from build123d import *

# Parameters (mm, degrees)
SKETCH1_R           = 15
BOSS_EXTRUDE1_DEPTH = 5
SKETCH2_R           = 19
SKETCH2_R_2         = 15
BOSS_EXTRUDE2_DEPTH = 40
SKETCH3_R           = 5
SKETCH3_R_2         = 15
BOSS_EXTRUDE4_DEPTH = 5
BOSS_EXTRUDE5_REACH = 62
SKETCH4_R           = 19
SKETCH5_R           = 10
CUT_EXTRUDE1_DEPTH  = 10
SKETCH6_R           = 5
CUT_EXTRUDE2_DEPTH  = 48
BOSS_EXTRUDE6_REACH = 62
SKETCH7_R           = 6
SKETCH8_R           = 2
CUT_EXTRUDE3_DEPTH  = 15


with BuildPart() as part:
    # Sketch1 → Boss-Extrude1 (new body)
    with BuildSketch(Plane(origin=(0, 0, 0), x_dir=(1, 0, 0), z_dir=(0, 1, 0))):
        with BuildLine():
            Line((-9.090909091, 17.814470857), (-30.909090909, 6.680426571))
            ThreePointArc((-30.909090909, 6.680426571), (-35, 0), (-30.909090909, -6.680426571))
            Line((-30.909090909, -6.680426571), (-9.090909091, -17.814470857))
            ThreePointArc((-9.090909091, -17.814470857), (0, -20), (9.090909091, -17.814470857))
            Line((9.090909091, -17.814470857), (30.909090909, -6.680426571))
            ThreePointArc((30.909090909, -6.680426571), (35, 0), (30.909090909, 6.680426571))
            Line((30.909090909, 6.680426571), (9.090909091, 17.814470857))
            ThreePointArc((9.090909091, 17.814470857), (0, 20), (-9.090909091, 17.814470857))
        make_face()
        Circle(SKETCH1_R, mode=Mode.SUBTRACT)
        with BuildLine():
            Line((-23.5, 2), (-24.035898385, 2))
            ThreePointArc((-24.035898385, 2), (-31.5, 0), (-24.035898385, -2))
            Line((-24.035898385, -2), (-23.5, -2))
            Line((-23.5, -2), (-19.5, -2))
            Line((-19.5, -2), (-19.5, 2))
            Line((-19.5, 2), (-23.5, 2))
        make_face(mode=Mode.SUBTRACT)
        with BuildLine():
            Line((23.5, 2), (24.035898385, 2))
            ThreePointArc((24.035898385, 2), (31.5, 0), (24.035898385, -2))
            Line((24.035898385, -2), (23.5, -2))
            Line((23.5, -2), (19.5, -2))
            Line((19.5, -2), (19.5, 2))
            Line((19.5, 2), (23.5, 2))
        make_face(mode=Mode.SUBTRACT)
    extrude(amount=BOSS_EXTRUDE1_DEPTH)

    # Sketch2 → Boss-Extrude2 (add)
    with BuildSketch(Plane(origin=(0, 5, 0), x_dir=(1, 0, 0), z_dir=(0, 1, 0))):
        Circle(SKETCH2_R)
        Circle(SKETCH2_R_2, mode=Mode.SUBTRACT)
    extrude(amount=BOSS_EXTRUDE2_DEPTH)

    # Sketch3 → Boss-Extrude4 (add)
    with BuildSketch(Plane(origin=(0, 45, 0), x_dir=(1, 0, 0), z_dir=(0, 1, 0))):
        with BuildLine():
            Line((9.090909091, -17.814470857), (30.909090909, -6.680426571))
            ThreePointArc((30.909090909, -6.680426571), (35, 0), (30.909090909, 6.680426571))
            Line((30.909090909, 6.680426571), (9.090909091, 17.814470857))
            ThreePointArc((9.090909091, 17.814470857), (0, 20), (-9.090909091, 17.814470857))
            Line((-9.090909091, 17.814470857), (-30.909090909, 6.680426571))
            ThreePointArc((-30.909090909, 6.680426571), (-35, 0), (-30.909090909, -6.680426571))
            Line((-30.909090909, -6.680426571), (-9.090909091, -17.814470857))
            ThreePointArc((-9.090909091, -17.814470857), (0, -20), (9.090909091, -17.814470857))
        make_face()
        with Locations((-27.5, 0)):
            Circle(SKETCH3_R, mode=Mode.SUBTRACT)
        with Locations((27.5, 0)):
            Circle(SKETCH3_R, mode=Mode.SUBTRACT)
        Circle(SKETCH3_R_2, mode=Mode.SUBTRACT)
    extrude(amount=BOSS_EXTRUDE4_DEPTH)

    # Sketch4 → Boss-Extrude5 (add, up to next)
    with BuildSketch(Plane.XY.offset(40), mode=Mode.PRIVATE) as boss_extrude5_sk1:
        with Locations((0, 25)):
            Circle(SKETCH4_R)
    boss_extrude5_tool1 = extrude(boss_extrude5_sk1.sketch, amount=-BOSS_EXTRUDE5_REACH, mode=Mode.PRIVATE) - part.part
    add(boss_extrude5_tool1.solids().sort_by_distance((0, 25, 40))[0])

    # Sketch5 → Cut-Extrude1 (cut)
    with BuildSketch(Plane.XY.offset(40)):
        with Locations((0, 25)):
            Circle(SKETCH5_R)
    extrude(amount=-CUT_EXTRUDE1_DEPTH, mode=Mode.SUBTRACT)

    # Sketch6 → Cut-Extrude2 (cut)
    with BuildSketch(Plane.XY.offset(30)):
        with Locations((0, 25)):
            Circle(SKETCH6_R)
    extrude(amount=-CUT_EXTRUDE2_DEPTH, mode=Mode.SUBTRACT)

    # Sketch7 → Boss-Extrude6 (add, up to next)
    with BuildSketch(Plane.XY.offset(-20), mode=Mode.PRIVATE) as boss_extrude6_sk1:
        with Locations((0, 25)):
            Circle(SKETCH7_R)
    boss_extrude6_tool1 = extrude(boss_extrude6_sk1.sketch, amount=BOSS_EXTRUDE6_REACH, mode=Mode.PRIVATE) - part.part
    add(boss_extrude6_tool1.solids().sort_by_distance((0, 25, -20))[0])

    # Sketch8 → Cut-Extrude3 (cut)
    with BuildSketch(Plane.XY.offset(40)):
        with Locations((0, 39.5)):
            Circle(SKETCH8_R)
        with Locations((12.557368355, 17.75)):
            Circle(SKETCH8_R)
        with Locations((-12.557368355, 17.75)):
            Circle(SKETCH8_R)
    extrude(amount=-CUT_EXTRUDE3_DEPTH, mode=Mode.SUBTRACT)


solid = part.part
Build history of the part. All positions in model axes, mm. A direction names the side the tool comes from. Give positions to 0.01 mm unless a question says otherwise; leave off trailing zeros. Order: outer loops, then holes, each group sorted by start corner. A loop starts at its lowest first (then second) coordinate and runs counter-clockwise, first axis right, second up. Notation, with made-up numbers: M 78.5,-37 L 114.5,-37 A27 ccw 114.5,-16 Z; hole C 55.5,60 d3. An arc over 180 degrees is marked long. Use one line per item in the form item = value.
Q1. Which spindle directions (+Z, -Z, +X, -X, +Y, -Y) get a long thin tool onto all of the face, cutting with end or side? Do faces 4 (the flat face through (-22, 2, -2)), 5 (the flat face through (-18.3, 5, 5.8)), 6 (the cylindrical face through (-1.302, 34.915, 35.07)). Say none if no direction does.
Conclusion:
face_4 = -Y
face_5 = none
face_6 = +Z
Q2. Slice it at D-D, the plane z = -8.5. Write the cut outline in (x, y).
Conclusion:
outline = M -27.34,0 L -12.36,0 L -12.36,50 L -27.34,50 L -27.34,45 L -16.99,45 L -16.99,5 L -27.34,5 Z; M 12.36,0 L 27.34,0 L 27.34,5 L 16.99,5 L 16.99,45 L 27.34,45 L 27.34,50 L 12.36,50 Z
Q3. Slice it at B-B, the plane z = 26.5. Write the cut outline in (x, y), and give its area (3 significant figures).
Conclusion:
outline = C 0,25 d38; hole C -12.56,17.75 d4; hole C 0,25 d10; hole C 0,39.5 d4; hole C 12.56,17.75 d4
area = 1,020 mm2
Q4. Pin check, flat tips, straight feed: P1, Ø10, axis at x = -1, z = -13, coming from the -Y side; P2, Ø5, axis at x = -22.5, y = 1.5, coming from the -Z side; P3, Ø3.5, axis at x = -12.56, y = 17.75, coming from the -Z side; P4, Ø2.5, axis at x = 0, y = 39.5, coming from the +Z side. Stop position of each tip, or through.
Conclusion:
P1 = 0
P2 = -12.25
P3 = -15.63
P4 = 25
Q5. Wall check: probe 1 along Y at (x, z) = (0, 35); probe 2 along X at (y, z) = (17.5, 0); probe 3 along Z at (x, y) = (0, 32). Give the ranges that are in metal, low to high.
Conclusion:
probe_1 = 6 to 15, 35 to 37.5, 41.5 to 44
probe_2 = -19 to -15, 15 to 19
probe_3 = -19 to -15, 15 to 30
Q6. Pull direction Y, two halves, no side cores. Call faces 1 (the cylindrical face through (-14.031, 19.102, 32.605)), 2 (the flat face through (-19.847, 2.465, -12.325)), 3 (the flat face through (0, 25, -18)): released by +Y, released by -Y, zero draft, split by the parting line, or undercut.
Conclusion:
face_1 = undercut
face_2 = zero draft
face_3 = undercut
Q7. Slice it at A-A, the plane x = 27.5. Write the cut outline in (y, z).
Conclusion:
outline = M 0,-8.42 L 5,-8.42 L 5,-4 L 0,-4 Z; M 0,4 L 5,4 L 5,8.42 L 0,8.42 Z; M 45,-8.42 L 50,-8.42 L 50,-5 L 45,-5 Z; M 45,5 L 50,5 L 50,8.42 L 45,8.42 Z
Q8. Slice it at C-C, the plane y = 33.5. Write the cut outline in (x, z).
Conclusion:
outline = M -16.99,8.5 A19 ccw long 16.99,8.5 L 16.99,40 L 5.27,40 L 5.27,30 L -5.27,30 L -5.27,40 L -16.99,40 Z; hole C 0,0 d30
